```python
from build123d import *

# Parameters (mm, degrees)
SKETCH1_R             = 4
BOSS_EXTRUDE1_DEPTH   = 5
BODY_MOVE_COPY1_ANGLE = 82.5


with BuildPart() as part:
    # Sketch1 → Boss-Extrude1 (new body)
    with BuildSketch(Plane(origin=(0, 0, 0), x_dir=(1, 0, 0), z_dir=(0, 1, 0))):
        with BuildLine():
            Line((17.104515265, -14.844249905), (183.104515265, -14.844249905))
            Line((183.104515265, -14.844249905), (202.418839623, -10.490300594))
            ThreePointArc((202.418839623, -10.490300594), (208.912700196, 6.687224641), (190.565681892, 5.896960314))
            ThreePointArc((190.565681892, 5.896960314), (183.998945909, -0.509119996), (175.127942725, -2.846894344))
            Line((175.127942725, -2.846894344), (24.726164692, -2.84688969))
            ThreePointArc((24.726164692, -2.84688969), (15.931189962, -0.551933774), (9.378890583, 5.747730981))
            ThreePointArc((9.378890583, 5.747730981), (-8.988354121, 6.341095346), (-2.269343204, -10.763367569))
            Line((-2.269343204, -10.763367569), (17.104515265, -14.844249905))
        make_face()
        Circle(SKETCH1_R, mode=Mode.SUBTRACT)
        with Locations((199.999855487, 0.240427049)):
            Circle(SKETCH1_R, mode=Mode.SUBTRACT)
    extrude(amount=BOSS_EXTRUDE1_DEPTH)


with BuildPart() as part_1:
    # Body-Move/Copy1: moved
    add(part.part.rotate(Axis((99.999927744, 2.5, 0), (0, 0, 1)), BODY_MOVE_COPY1_ANGLE))


solid = part_1.part
```
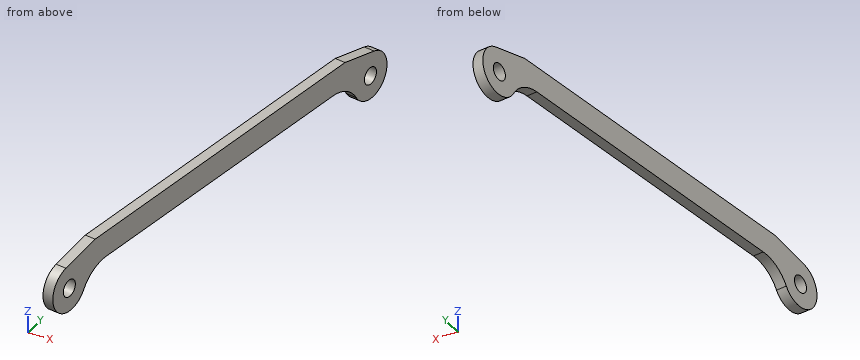
CAD build for the part. Positions are in the model's coordinates, mm. Give positions to 0.01 mm unless a question says otherwise; leave off trailing zeros. Write each loop counter-clockwise with the first axis right and the second up, starting at its lowest first coordinate (ties: lowest second). Pieces come first, ordered by that corner, then holes. Notation, with made-up numbers: M 81,-22 L 118,-22 A25 cw 118,1 Z; hole C 33.25,66.5 d11. An arc over 180 degrees is marked long. Return JSON: item names as keys, results as strings. Group by question number.
(1) Band-saw the part on B-B (y = -54.5). Give the cut face in (x, z), and give its area (3 significant figures).
(2) Drill centre lines: L1, parallel to X at y = -18, z = 10.75; L2, parallel to Z at x = 96, y = -24; L3, parallel to X at y = 27, z = 3. Where is each one in solid material? Low to high. Write a range as [from, to].
(3) Band-saw the part on C-C (x = 100.5). Give the cut face in (y, z).
(4) Band-saw the part on A-A (z = -7.75). Give the cut face in (x, y).
(5) Flat gauge pins, fed straight in: pin 1 Ø6 at (y, z) = (88.5, 5) entering from -X; pin 2 Ø1 at (y, z) = (-2, 8.5) entering from +X; pin 3 Ø12 at (x, y) = (101, 69) entering from -Z. Where does each tip first touch, or does it go through?
Entries:
{
 "1": {"outline": "M 89.97,2.85 L 95.02,2.85 L 95.02,14.84 L 89.97,14.84 Z", "area": "60.5 mm^2"},
 "2": {"L1": "x = [94.78, 99.82]", "L2": "z = [2.85, 14.84]", "L3": "x = [100.7, 105.75]"},
 "3": {"outline": "M -12.85,2.85 L 25.45,2.85 L 25.45,14.84 L -12.85,14.84 Z"},
 "4": {"outline": "M 83.45,-104.06 L 88.41,-104.71 L 90.44,-89.23 L 85.49,-88.58 Z; M 109.52,94 L 114.48,93.35 L 116.58,109.29 L 111.62,109.94 Z"},
 "5": {"pin 1": "stops at x = 108.41", "pin 2": "stops at x = 101.99", "pin 3": "stops at z = 2.85"}
}
